Could you check a few things on this drawing? It's one solid part, dimensions in mm from its lowest x, y, z. Round coordinates to 2 decimals unless told otherwise and drop trailing zeros. Write each loop counter-clockwise with the first axis right and the second up, starting at its lowest first coordinate (ties: lowest second). Pieces come first, ordered by that corner, then holes. Notation, with made-up numbers: (19, 25) - (41, 25) arc R35 cw to (41, 60) - close; hole circle Ø6 at (74, 74.25). An arc over 180 degrees is marked (long way). Write item = value, one per line. Start each with the question number.
Item 1: For P1, Ø1.9, axis at x = 150, z = 2, coming from the -Y side; P2, Ø1.9, axis at y = 124, z = 3.5, coming from the -X side; P3, Ø2, axis at y = 302, z = 3, coming from the +X side (1 decimal), each with a flat end and sliding along its axis, tell me the tip position at first contact or that it passes through.
Item 2: If I drill on line 1 along Y through (x, z) = (107.5, 2.5) (1 decimal); line 2 along Y through (x, z) = (43, 4.5); line 3 along X through (y, z) = (85, 3.25) (1 decimal), over which ranges is the centre line in solid material (lowest first)? Write a range as [from, to].
Item 3: If we section it at A-A (x = 54): Please give me the cut outline in (y, z).
Item 4: If we section it at D-D (y = 157.5): Please give me the cut outline in (x, z).
Item 5: If we section it at C-C (x = 28): Please give me the cut outline in (y, z).
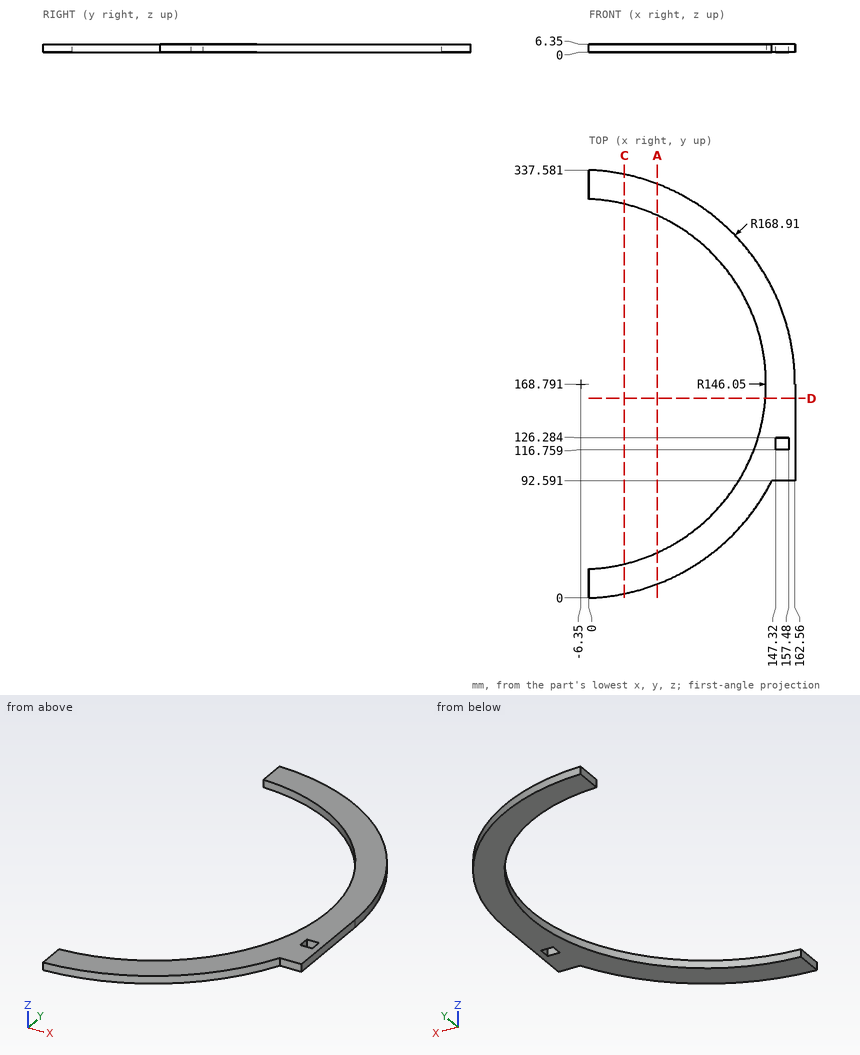
Reply:
q1.P1 = 92.59
q1.P2 = 132.35
q1.P3 = 98.8
q2.line_1 = [44, 77.3], [260.3, 293.6]
q2.line_2 = [7.25, 31.33], [306.25, 330.33]
q2.line_3 = [113.3, 140.3]
q3.outline = (11.03, 0) - (35.79, 0) - (35.79, 6.35) - (11.03, 6.35) - close; (301.79, 0) - (326.55, 0) - (326.55, 6.35) - (301.79, 6.35) - close
q4.outline = (139.26, 0) - (162.56, 0) - (162.56, 6.35) - (139.26, 6.35) - close
q5.outline = (3.41, 0) - (26.84, 0) - (26.84, 6.35) - (3.41, 6.35) - close; (310.74, 0) - (334.17, 0) - (334.17, 6.35) - (310.74, 6.35) - close
